```python
from build123d import *

# Parameters (mm, degrees)
F1_DEPTH      = 100
F3_DEPTH      = 25
F3_DEPTH_BACK = 25
F4_SIZE       = 2.90999
F5_SIZE       = 2.90999
F7_DEPTH      = 6.25
F8_SIZE       = 1
F9_C1_SIZE    = 0.5
F9_C2_SIZE    = 0.5
F9_C3_SIZE    = 0.5
F9_C4_SIZE    = 0.5
F9_C5_SIZE    = 0.5
F9_C6_SIZE    = 0.5
F9_C7_SIZE    = 0.5
F9_C8_SIZE    = 0.5
F9_C9_SIZE    = 0.5
F9_C10_SIZE   = 0.5
F9_C11_SIZE   = 0.5
F9_C12_SIZE   = 0.5
F9_C13_SIZE   = 0.5
F9_C14_SIZE   = 0.5
F9_C15_SIZE   = 0.5
F9_C16_SIZE   = 0.5
F9_C17_SIZE   = 0.5
F9_C18_SIZE   = 0.5
F9_C19_SIZE   = 0.5
F9_C20_SIZE   = 0.5
F9_C21_SIZE   = 0.5
F9_C22_SIZE   = 0.5
F9_C23_SIZE   = 0.5
F9_C24_SIZE   = 0.5


# Not quite as in the source:
# - a fillet or chamfer is up to 0.001 mm smaller than in the source, because OpenCascade refuses the exact size


with BuildPart() as f1:
    # F0 (on Top) → F1 (new body)
    with BuildSketch(Plane.XY):
        Polygon((0, 2.91), (0, 0), (4.5, 0), (6, 1.5), (12, 1.5), (13.5, 0), (18, 0), (18, 2.91), (15.2, 2.91), (15.2, 6.91), (2.8, 6.91), (2.8, 2.91), align=None)
    extrude(amount=F1_DEPTH)

    # F2 (on Right) → F3 (cut, two sides)
    with BuildSketch(Plane.YZ) as f3_sk:
        Polygon((-0.9837878169, 0), (0, 0), (0, 35), (1.5, 36.5), (1.5, 40), (0, 41.5), (0, 66.5), (1.5, 68), (1.5, 71.5), (0, 73), (0, 100.0014618039), (-0.9837878169, 100.0014618039), align=None)
    extrude(amount=-F3_DEPTH, mode=Mode.SUBTRACT)
    extrude(f3_sk.sketch, amount=F3_DEPTH_BACK, mode=Mode.SUBTRACT)

    # F4 (size 2.91 in the source; OpenCascade refuses exactly that, so slightly less here)
    f4_edges = [f1.edges().sort_by_distance(p)[0] for p in [
        (2.25, 0, 0),
    ]]
    chamfer(f4_edges, length=F4_SIZE)

    # F5 (size 2.91 in the source; OpenCascade refuses exactly that, so slightly less here)
    f5_edges = [f1.edges().sort_by_distance(p)[0] for p in [
        (15.75, 0, 100),
    ]]
    chamfer(f5_edges, length=F5_SIZE)

    # F6 (on Front) → F7 (cut)
    with BuildSketch(Plane.XZ):
        Polygon((6.375, 14), (9, 14), (11.625, 14), (11.625, 19.5), (6.375, 19.5), align=None)
    extrude(amount=-F7_DEPTH, mode=Mode.SUBTRACT)

    # F8
    f8_edges = [f1.edges().sort_by_distance(p)[0] for p in [
        (9, 1.5, 14),
        (9, 1.5, 19.5),
    ]]
    chamfer(f8_edges, length=F8_SIZE)

    # F9: chamfer of 0.5 on 28 edges, made by hand

    # F9_c1
    f9_c1_edges = [f1.edges().sort_by_distance(p)[0] for p in [
        (18, 2.91, 50),
    ]]
    chamfer(f9_c1_edges, length=F9_C1_SIZE)

    # F9_c2
    f9_c2_edges = [f1.edges().sort_by_distance(p)[0] for p in [
        (0, 2.91, 50),
    ]]
    chamfer(f9_c2_edges, length=F9_C2_SIZE)

    # F9_c3
    f9_c3_edges = [f1.edges().sort_by_distance(p)[0] for p in [
        (18, 0, 18.954995),
    ]]
    chamfer(f9_c3_edges, length=F9_C3_SIZE)

    # F9_c4
    f9_c4_edges = [f1.edges().sort_by_distance(p)[0] for p in [
        (0, 0, 18.954995),
    ]]
    chamfer(f9_c4_edges, length=F9_C4_SIZE)

    # F9_c5
    f9_c5_edges = [f1.edges().sort_by_distance(p)[0] for p in [
        (18, 0, 54),
    ]]
    chamfer(f9_c5_edges, length=F9_C5_SIZE)

    # F9_c6
    f9_c6_edges = [f1.edges().sort_by_distance(p)[0] for p in [
        (0, 0, 54),
    ]]
    chamfer(f9_c6_edges, length=F9_C6_SIZE)

    # F9_c7
    f9_c7_edges = [f1.edges().sort_by_distance(p)[0] for p in [
        (0, 0, 85.045005),
    ]]
    chamfer(f9_c7_edges, length=F9_C7_SIZE)

    # F9_c8
    f9_c8_edges = [f1.edges().sort_by_distance(p)[0] for p in [
        (18, 0, 85.045005),
    ]]
    chamfer(f9_c8_edges, length=F9_C8_SIZE)

    # F9_c9
    f9_c9_edges = [f1.edges().sort_by_distance(p)[0] for p in [
        (18, 1.455, 1.45499),
    ]]
    chamfer(f9_c9_edges, length=F9_C9_SIZE)

    # F9_c10
    f9_c10_edges = [f1.edges().sort_by_distance(p)[0] for p in [
        (0, 1.455, 1.45499),
    ]]
    chamfer(f9_c10_edges, length=F9_C10_SIZE)

    # F9_c11
    f9_c11_edges = [f1.edges().sort_by_distance(p)[0] for p in [
        (18, 1.455, 98.54501),
    ]]
    chamfer(f9_c11_edges, length=F9_C11_SIZE)

    # F9_c12
    f9_c12_edges = [f1.edges().sort_by_distance(p)[0] for p in [
        (0, 1.455, 98.54501),
    ]]
    chamfer(f9_c12_edges, length=F9_C12_SIZE)

    # F9_c13
    f9_c13_edges = [f1.edges().sort_by_distance(p)[0] for p in [
        (18, 1.5, 69.75),
    ]]
    chamfer(f9_c13_edges, length=F9_C13_SIZE)

    # F9_c14
    f9_c14_edges = [f1.edges().sort_by_distance(p)[0] for p in [
        (0, 1.5, 69.75),
    ]]
    chamfer(f9_c14_edges, length=F9_C14_SIZE)

    # F9_c15
    f9_c15_edges = [f1.edges().sort_by_distance(p)[0] for p in [
        (18, 1.5, 38.25),
    ]]
    chamfer(f9_c15_edges, length=F9_C15_SIZE)

    # F9_c16
    f9_c16_edges = [f1.edges().sort_by_distance(p)[0] for p in [
        (0, 1.5, 38.25),
    ]]
    chamfer(f9_c16_edges, length=F9_C16_SIZE)

    # F9_c17
    f9_c17_edges = [f1.edges().sort_by_distance(p)[0] for p in [
        (18, 1, 36),
    ]]
    chamfer(f9_c17_edges, length=F9_C17_SIZE)

    # F9_c18
    f9_c18_edges = [f1.edges().sort_by_distance(p)[0] for p in [
        (18, 1, 40.5),
    ]]
    chamfer(f9_c18_edges, length=F9_C18_SIZE)

    # F9_c19
    f9_c19_edges = [f1.edges().sort_by_distance(p)[0] for p in [
        (0, 1, 72),
    ]]
    chamfer(f9_c19_edges, length=F9_C19_SIZE)

    # F9_c20
    f9_c20_edges = [f1.edges().sort_by_distance(p)[0] for p in [
        (18, 1, 72),
    ]]
    chamfer(f9_c20_edges, length=F9_C20_SIZE)

    # F9_c21
    f9_c21_edges = [f1.edges().sort_by_distance(p)[0] for p in [
        (18, 1, 67.5),
    ]]
    chamfer(f9_c21_edges, length=F9_C21_SIZE)

    # F9_c22
    f9_c22_edges = [f1.edges().sort_by_distance(p)[0] for p in [
        (0, 1, 36),
    ]]
    chamfer(f9_c22_edges, length=F9_C22_SIZE)

    # F9_c23
    f9_c23_edges = [f1.edges().sort_by_distance(p)[0] for p in [
        (0, 1, 40.5),
    ]]
    chamfer(f9_c23_edges, length=F9_C23_SIZE)

    # F9_c24
    f9_c24_edges = [f1.edges().sort_by_distance(p)[0] for p in [
        (0, 1, 67.5),
    ]]
    chamfer(f9_c24_edges, length=F9_C24_SIZE)


solid = f1.part
```
Source: CAD feature listing. Evaluate the final solid. Frame: model axes, mm. A direction names the side the tool comes from. Coordinates: 2 decimals unless noted, no trailing zeros. Loops run counter-clockwise (first coordinate to the right, second up) from the corner with the lowest first, then second, coordinate; pieces in that order, holes last. Notation, with made-up numbers: (57, 4.5) - (103, 4.5) arc R11 ccw to (103, 9.5) - close; hole circle Ø8 at (2.5, -11.5). An arc over 180 degrees is marked (long way). Answer as CSV lines item,"result".
1. Section B-B (z = 18.5). Return loops of the section in (x, y) (3 decimals), then the cut area to 3 significant figures.
Established:
outline,"(0, 0.5) - (0.5, 0) - (4.5, 0) - (6, 1.5) - (6.375, 1.5) - (6.375, 6.25) - (11.625, 6.25) - (11.625, 1.5) - (12, 1.5) - (13.5, 0) - (17.5, 0) - (18, 0.5) - (18, 2.41) - (17.5, 2.91) - (15.2, 2.91) - (15.2, 6.91) - (2.8, 6.91) - (2.8, 2.91) - (0.5, 2.91) - (0, 2.41) - close"
area,"65.3 mm2"
2. Reachability of faces 4 (the flat face through (15.2, 5, 49)), 5 (the flat face through (0.25, 1.01, 35.66)), 6 (the flat face through (6.375, 4, 17)), 7 (the flat face through (2, 2.91, 49)), 8 (the flat face through (17.754, 0.991, 67.132)) from +Z, -Z, +X, -X, +Y, -Y: full face, straight path, thin tool, end or side. Return the list, or none.
Established:
face 4,"+Z, -Z, +X, +Y"
face 5,"-X, -Y"
face 6,"-Y"
face 7,"+Z, -Z, -X, +Y"
face 8,"+X, -Y"
3. Ray query, line 1 (Z direction, x = 15.75, y = 1); line 2 (Y direction, x = 1.5, z = 28); line 3 (X direction, y = 6.5, z = 10.5). Return the intervals inside material, ascending.
Established:
line 1,"z = 1.91 to 36, 40.5 to 67.5, 72 to 98.09"
line 2,"y = 0 to 2.91"
line 3,"x = 2.8 to 15.2"
4. Contact query for flat-ended pins moving along their axis: pin 1 (4 mm diameter, centred on x = 9, z = 74, fed in from -Y); pin 2 (1.2 mm diameter, centred on x = 16, z = 37, fed in from +Y); pin 3 (1.2 mm diameter, centred on y = 4.5, z = 69, fed in from -X); pin 4 (1 mm diameter, centred on x = 8, y = 5, fed in from -Z). Output: stop coordinate, or through.
Established:
pin 1,"stops at y = 1.5"
pin 2,"stops at y = 2.91"
pin 3,"stops at x = 2.8"
pin 4,"stops at z = 0"
5. Mould query, pull axis X, two halves, no side actions, for faces 1 (the flat face through (0.25, 1.01, 67.16)), 2 (the flat face through (9, 4, 14)), 3 (the flat face through (18, 1, 49)). Classes: released by +X, released by -X, zero draft, split by the parting line, or undercut.
Established:
face 1,"released by -X"
face 2,"undercut"
face 3,"released by +X"
6. Section C-C (x = 8.5). Return loops of the section in (y, z), then the cut area to 3 significant figures.
Established:
outline,"(1.5, 1.41) - (2.91, 0) - (6.91, 0) - (6.91, 100) - (2.91, 100) - (1.5, 98.59) - (1.5, 20.5) - (2.5, 19.5) - (6.25, 19.5) - (6.25, 14) - (2.5, 14) - (1.5, 13) - close"
area,"512 mm2"
7. Section A-A (y = 5.25). Return loops of the section in (x, z) (3 decimals).
Established:
outline,"(2.8, 0) - (15.2, 0) - (15.2, 100) - (2.8, 100) - close; hole (6.375, 14) - (11.625, 14) - (11.625, 19.5) - (6.375, 19.5) - close"
